Can you work these out from the drawing? Everything is in mm from the part's minimum corner. A direction names the side the tool comes from. Give positions to 0.01 mm unless a question says otherwise; leave off trailing zeros. Loops run counter-clockwise (first coordinate to the right, second up) from the corner with the lowest first, then second, coordinate; pieces in that order, holes last.
Q1. If we section it at B-B (z = 9.5): Please give me the cut outline in (x, y), plus the area to 3 significant figures.
Q2. If we section it at C-C (z = 3): Please give me the cut outline in (x, y).
Q3. We'd pull the mould along X, two halves only. Please class the marked faces 1, 2 and 3: +X half, -X half, draft (parallel to the pull), parting line (faces both ways), or undercut.
Q4. For the marked faces 4, 5 and 6, which set-ups out of +Z, -Z, +X, -X, +Y, -Y let a thin tool reach every point of the face, with its end or its side?
Q5. Will these pins go through, and if not, where does the flat tip stop? P1, Ø1, axis at x = 20.5, z = 9.5, coming from the -Y side; P2, Ø2.5, axis at x = 18.5, z = 6, coming from the -Y side; P3, Ø0.9, axis at x = 6, z = 9, coming from the +Y side.
Q6. If we section it at D-D (y = 7.5): Please give me the cut outline in (x, z), plus the area to 3 significant figures.
Q7. If we section it at A-A (y = 16): Please give me the cut outline in (x, z).
Q8. I need wall thicknesses on line 1 (Z direction, x = 6.1, y = 16.1); line 2 (X direction, y = 8, z = 11); line 3 (Y direction, x = 4, z = 9). Which ranges of each line are inside material? Lowest first, please.
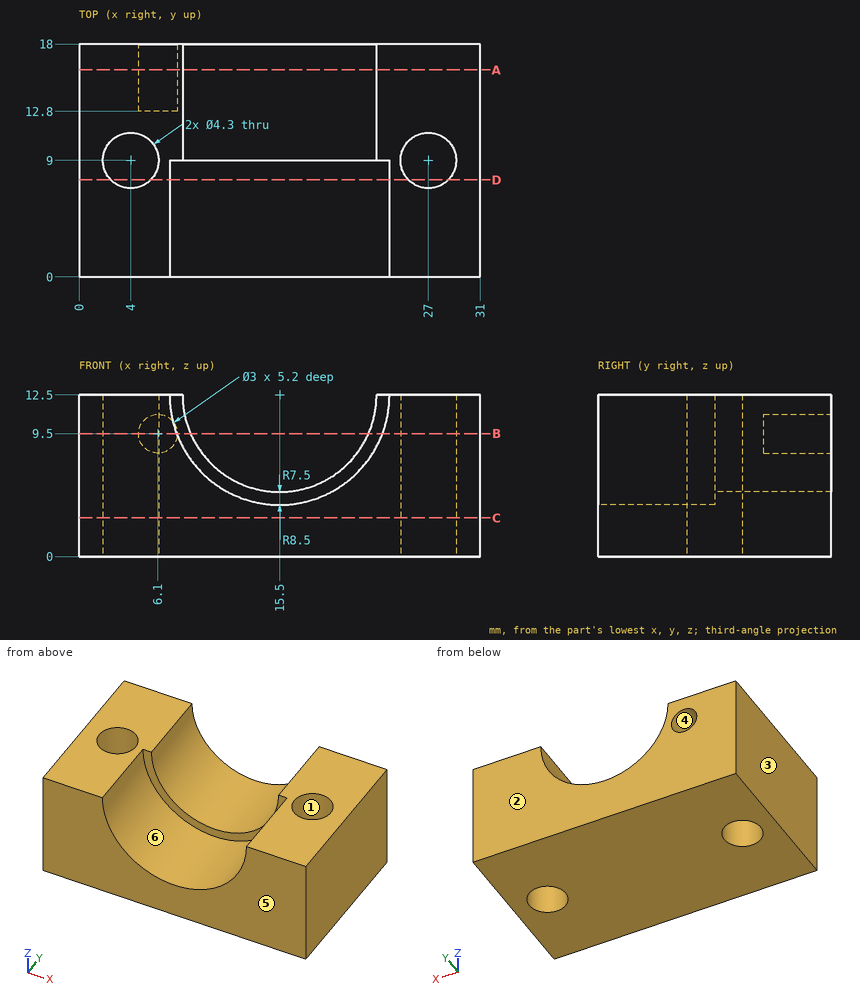
Check sheet entries:
1. outline: (0, 0) - (7.55, 0) - (7.55, 9) - (8.63, 9) - (8.63, 18) - (7.6, 18) - (7.6, 12.8) - (4.6, 12.8) - (4.6, 18) - (0, 18) - close; (22.37, 9) - (23.45, 9) - (23.45, 0) - (31, 0) - (31, 18) - (22.37, 18) - close; hole circle Ø4.3 at (4, 9); hole circle Ø4.3 at (27, 9)
1. area: 246 mm2
2. outline: (0, 0) - (31, 0) - (31, 18) - (0, 18) - close; hole circle Ø4.3 at (4, 9); hole circle Ø4.3 at (27, 9)
3. face 1: undercut
3. face 2: draft
3. face 3: -X half
4. face 4: +Y
4. face 5: +Z, -Z, +X, -X, -Y
4. face 6: +Z, -Y
5. P1: passes through
5. P2: stops at y = 9
5. P3: stops at y = 12.8
6. outline: (0, 0) - (2.46, 0) - (2.46, 12.5) - (0, 12.5) - close; (5.54, 0) - (25.46, 0) - (25.46, 12.5) - (24, 12.5) arc R8.5 cw to (7, 12.5) - (5.54, 12.5) - close; (28.54, 0) - (31, 0) - (31, 12.5) - (28.54, 12.5) - close
6. area: 197 mm2
7. outline: (0, 0) - (31, 0) - (31, 12.5) - (23, 12.5) arc R7.5 cw to (8, 12.5) - (0, 12.5) - close; hole circle Ø3 at (6.1, 9.5)
8. line 1: z = 0 to 8, 11 to 12.5
8. line 2: x = 0 to 2.1, 5.9 to 7.13, 23.87 to 25.1, 28.9 to 31
8. line 3: y = 0 to 6.85, 11.15 to 18
